Could you check a few things on this model? Use its own coordinates, in mm. A direction names the side the tool comes from. Round coordinates to 2 decimals unless told otherwise and drop trailing zeros. Order: outer loops, then holes, each group sorted by start corner. A loop starts at its lowest first (then second) coordinate and runs counter-clockwise, first axis right, second up. Notation, with made-up numbers: (74.5, 89) - (87.5, 89) arc R21 cw to (87.5, 124) - close; hole circle Ø4 at (25.25, 54.25). An arc over 180 degrees is marked (long way). Use one line per item in the form item = value.
from build123d import *

# Parameters (mm, degrees)
BOSS_EXTRUDE1_DEPTH = 26
FILLET1_R           = 2.5
CUT_EXTRUDE1_REACH  = 76.051
SKETCH2_R           = 3
CUT_EXTRUDE2_REACH  = 73.261
SKETCH3_R           = 3
CUT_EXTRUDE3_REACH  = 90.154
SKETCH4_R           = 3
SKETCH4_W           = 12
SKETCH4_H           = 20
BOSS_EXTRUDE2_DEPTH = 3
FILLET2_R           = 3.5


with BuildPart() as part:
    # Sketch1 → Boss-Extrude1 (new body)
    with BuildSketch(Plane(origin=(0, 0, 0), x_dir=(1, 0, 0), z_dir=(0, 1, 0))):
        Polygon((-55.080799194, 36.198206666), (23.167912006, 36.198206666), (-15.956443594, -31.567165046), align=None)
        Polygon((-51.616697579, 34.198206666), (19.703810391, 34.198206666), (-15.956443594, -27.567165046), align=None, mode=Mode.SUBTRACT)
    extrude(amount=BOSS_EXTRUDE1_DEPTH)

    # Fillet1
    fillet1_edges = [part.edges().sort_by_distance(p)[0] for p in [
        (-51.616697579, 13, -34.198206666),
        (-15.956443594, 13, 27.567165046),
        (19.703810391, 13, -34.198206666),
        (-55.080799194, 13, -36.198206666),
        (23.167912006, 13, -36.198206666),
        (-15.956443594, 13, 31.567165046),
    ]]
    fillet(fillet1_edges, radius=FILLET1_R)

    # Sketch2 → Cut-Extrude1 (cut, up to next)
    with BuildSketch(Plane(origin=(-25.636316123, 0, 14.801134015), x_dir=(0.49999999999999806, 0, 0.8660254037844397), z_dir=(-0.8660254037844397, 0, 0.49999999999999806)), mode=Mode.PRIVATE) as cut_extrude1_sk1:
        Polygon((3.632503749, 4.258248906), (-8.367496251, 8.741751094), (-8.367496251, 3), (3.632503749, 3), align=None)
    cut_extrude1_tool1 = extrude(cut_extrude1_sk1.sketch, amount=-CUT_EXTRUDE1_REACH, mode=Mode.PRIVATE) & part.part
    # Sketch2 → Cut-Extrude1 (cut, up to next)
    with BuildSketch(Plane(origin=(-25.636316123, 0, 14.801134015), x_dir=(0.49999999999999806, 0, 0.8660254037844397), z_dir=(-0.8660254037844397, 0, 0.49999999999999806)), mode=Mode.PRIVATE) as cut_extrude1_sk2:
        Polygon((-8.367496251, 13), (-8.367496251, 8.741751094), (3.632503749, 4.258248906), (3.632503749, 13), align=None)
    cut_extrude1_tool2 = extrude(cut_extrude1_sk2.sketch, amount=-CUT_EXTRUDE1_REACH, mode=Mode.PRIVATE) & part.part
    # Sketch2 → Cut-Extrude1 (cut, up to next)
    with BuildSketch(Plane(origin=(-25.636316123, 0, 14.801134015), x_dir=(0.49999999999999806, 0, 0.8660254037844397), z_dir=(-0.8660254037844397, 0, 0.49999999999999806)), mode=Mode.PRIVATE) as cut_extrude1_sk3:
        Polygon((3.632503749, 21.741751094), (-8.367496251, 17.258248906), (-8.367496251, 13), (3.632503749, 13), align=None)
    cut_extrude1_tool3 = extrude(cut_extrude1_sk3.sketch, amount=-CUT_EXTRUDE1_REACH, mode=Mode.PRIVATE) & part.part
    # Sketch2 → Cut-Extrude1 (cut, up to next)
    with BuildSketch(Plane(origin=(-25.636316123, 0, 14.801134015), x_dir=(0.49999999999999806, 0, 0.8660254037844397), z_dir=(-0.8660254037844397, 0, 0.49999999999999806)), mode=Mode.PRIVATE) as cut_extrude1_sk4:
        Polygon((-8.367496251, 23), (-8.367496251, 17.258248906), (3.632503749, 21.741751094), (3.632503749, 23), align=None)
    cut_extrude1_tool4 = extrude(cut_extrude1_sk4.sketch, amount=-CUT_EXTRUDE1_REACH, mode=Mode.PRIVATE) & part.part
    # Sketch2 → Cut-Extrude1 (cut, up to next)
    with BuildSketch(Plane(origin=(-25.636316123, 0, 14.801134015), x_dir=(0.49999999999999806, 0, 0.8660254037844397), z_dir=(-0.8660254037844397, 0, 0.49999999999999806)), mode=Mode.PRIVATE) as cut_extrude1_sk5:
        with Locations((-37.161724832, 13)):
            Circle(SKETCH2_R)
    cut_extrude1_tool5 = extrude(cut_extrude1_sk5.sketch, amount=-CUT_EXTRUDE1_REACH, mode=Mode.PRIVATE) & part.part
    add(cut_extrude1_tool1.solids().sort_by_distance((-27.460565, 4.989307, 11.641443))[0], mode=Mode.SUBTRACT)
    add(cut_extrude1_tool2.solids().sort_by_distance((-26.475179, 9.621142, 13.34818))[0], mode=Mode.SUBTRACT)
    add(cut_extrude1_tool3.solids().sort_by_distance((-26.475179, 16.378858, 13.34818))[0], mode=Mode.SUBTRACT)
    add(cut_extrude1_tool4.solids().sort_by_distance((-27.460565, 21.010693, 11.641443))[0], mode=Mode.SUBTRACT)
    add(cut_extrude1_tool5.solids().sort_by_distance((-44.217179, 13, -17.381864))[0], mode=Mode.SUBTRACT)

    # Sketch3 → Cut-Extrude2 (cut, up to next)
    with BuildSketch(Plane(origin=(1.701650732, 0, 0.982448508), x_dir=(0.5000000000000041, 0, -0.8660254037844364), z_dir=(0.8660254037844364, 0, 0.5000000000000041)), mode=Mode.PRIVATE) as cut_extrude2_sk1:
        Polygon((15.205281238, 13), (15.205281238, 8.741751094), (27.205281238, 4.258248906), (27.205281238, 13), align=None)
    cut_extrude2_tool1 = extrude(cut_extrude2_sk1.sketch, amount=-CUT_EXTRUDE2_REACH, mode=Mode.PRIVATE) & part.part
    # Sketch3 → Cut-Extrude2 (cut, up to next)
    with BuildSketch(Plane(origin=(1.701650732, 0, 0.982448508), x_dir=(0.5000000000000041, 0, -0.8660254037844364), z_dir=(0.8660254037844364, 0, 0.5000000000000041)), mode=Mode.PRIVATE) as cut_extrude2_sk2:
        Polygon((27.205281238, 4.258248906), (15.205281238, 8.741751094), (15.205281238, 3), (27.205281238, 3), align=None)
    cut_extrude2_tool2 = extrude(cut_extrude2_sk2.sketch, amount=-CUT_EXTRUDE2_REACH, mode=Mode.PRIVATE) & part.part
    # Sketch3 → Cut-Extrude2 (cut, up to next)
    with BuildSketch(Plane(origin=(1.701650732, 0, 0.982448508), x_dir=(0.5000000000000041, 0, -0.8660254037844364), z_dir=(0.8660254037844364, 0, 0.5000000000000041)), mode=Mode.PRIVATE) as cut_extrude2_sk3:
        Polygon((27.205281238, 21.741751094), (15.205281238, 17.258248906), (15.205281238, 13), (27.205281238, 13), align=None)
    cut_extrude2_tool3 = extrude(cut_extrude2_sk3.sketch, amount=-CUT_EXTRUDE2_REACH, mode=Mode.PRIVATE) & part.part
    # Sketch3 → Cut-Extrude2 (cut, up to next)
    with BuildSketch(Plane(origin=(1.701650732, 0, 0.982448508), x_dir=(0.5000000000000041, 0, -0.8660254037844364), z_dir=(0.8660254037844364, 0, 0.5000000000000041)), mode=Mode.PRIVATE) as cut_extrude2_sk4:
        Polygon((15.205281238, 23), (15.205281238, 17.258248906), (27.205281238, 21.741751094), (27.205281238, 23), align=None)
    cut_extrude2_tool4 = extrude(cut_extrude2_sk4.sketch, amount=-CUT_EXTRUDE2_REACH, mode=Mode.PRIVATE) & part.part
    # Sketch3 → Cut-Extrude2 (cut, up to next)
    with BuildSketch(Plane(origin=(1.701650732, 0, 0.982448508), x_dir=(0.5000000000000041, 0, -0.8660254037844364), z_dir=(0.8660254037844364, 0, 0.5000000000000041)), mode=Mode.PRIVATE) as cut_extrude2_sk5:
        with Locations((-13.588947343, 13)):
            Circle(SKETCH3_R)
    cut_extrude2_tool5 = extrude(cut_extrude2_sk5.sketch, amount=-CUT_EXTRUDE2_REACH, mode=Mode.PRIVATE) & part.part
    add(cut_extrude2_tool1.solids().sort_by_distance((12.649176, 9.621142, -17.979222))[0], mode=Mode.SUBTRACT)
    add(cut_extrude2_tool2.solids().sort_by_distance((11.663791, 4.989307, -16.272485))[0], mode=Mode.SUBTRACT)
    add(cut_extrude2_tool3.solids().sort_by_distance((12.649176, 16.378858, -17.979222))[0], mode=Mode.SUBTRACT)
    add(cut_extrude2_tool4.solids().sort_by_distance((11.663791, 21.010693, -16.272485))[0], mode=Mode.SUBTRACT)
    add(cut_extrude2_tool5.solids().sort_by_distance((-5.092823, 13, 12.750822))[0], mode=Mode.SUBTRACT)

    # Sketch4 → Cut-Extrude3 (cut, up to next)
    with BuildSketch(Plane(origin=(0, 0, -36.198206666), x_dir=(-1, 0, 0), z_dir=(0, 0, -1)), mode=Mode.PRIVATE) as cut_extrude3_sk1:
        with Locations((-1.440670696, 13)):
            Circle(SKETCH4_R)
    cut_extrude3_tool1 = extrude(cut_extrude3_sk1.sketch, amount=-CUT_EXTRUDE3_REACH, mode=Mode.PRIVATE) & part.part
    # Sketch4 → Cut-Extrude3 (cut, up to next)
    with BuildSketch(Plane(origin=(0, 0, -36.198206666), x_dir=(-1, 0, 0), z_dir=(0, 0, -1)), mode=Mode.PRIVATE) as cut_extrude3_sk2:
        with Locations((15.956443594, 13)):
            Rectangle(SKETCH4_W, SKETCH4_H)
    cut_extrude3_tool2 = extrude(cut_extrude3_sk2.sketch, amount=-CUT_EXTRUDE3_REACH, mode=Mode.PRIVATE) & part.part
    # Sketch4 → Cut-Extrude3 (cut, up to next)
    with BuildSketch(Plane(origin=(0, 0, -36.198206666), x_dir=(-1, 0, 0), z_dir=(0, 0, -1)), mode=Mode.PRIVATE) as cut_extrude3_sk3:
        with Locations((33.353557885, 13)):
            Rectangle(SKETCH4_W, SKETCH4_H)
    cut_extrude3_tool3 = extrude(cut_extrude3_sk3.sketch, amount=-CUT_EXTRUDE3_REACH, mode=Mode.PRIVATE) & part.part
    add(cut_extrude3_tool1.solids().sort_by_distance((1.440671, 13, -36.198207))[0], mode=Mode.SUBTRACT)
    add(cut_extrude3_tool2.solids().sort_by_distance((-15.956444, 13, -36.198207))[0], mode=Mode.SUBTRACT)
    add(cut_extrude3_tool3.solids().sort_by_distance((-33.353558, 13, -36.198207))[0], mode=Mode.SUBTRACT)

    # Sketch5 → Boss-Extrude2 (add)
    with BuildSketch(Plane.XZ):
        with BuildLine():
            Line((-17.038975349, -12.984749429), (-33.786570587, -3.31552081))
            Line((-33.786570587, -3.31552081), (-34.786570587, -5.047571617))
            Line((-34.786570587, -5.047571617), (-17.956443594, -14.764449967))
            Line((-17.956443594, -14.764449967), (-17.956443594, -34.198206666))
            Line((-17.956443594, -34.198206666), (-15.956443594, -34.198206666))
            Line((-15.956443594, -34.198206666), (-15.956443594, -14.859749429))
            ThreePointArc((-15.956443594, -14.859749429), (-17.038975349, -14.234749429), (-17.038975349, -12.984749429))
        make_face()
        with BuildLine():
            Line((-32.786570587, -1.583470002), (-33.786570587, -3.31552081))
            Line((-33.786570587, -3.31552081), (-17.038975349, -12.984749429))
            ThreePointArc((-17.038975349, -12.984749429), (-15.956443594, -12.359749429), (-14.873911839, -12.984749429))
            Line((-14.873911839, -12.984749429), (1.873683398, -3.31552081))
            Line((1.873683398, -3.31552081), (0.873683398, -1.583470002))
            Line((0.873683398, -1.583470002), (-15.956443594, -11.300348352))
            Line((-15.956443594, -11.300348352), (-32.786570587, -1.583470002))
        make_face()
        with BuildLine():
            Line((1.873683398, -3.31552081), (-14.873911839, -12.984749429))
            ThreePointArc((-14.873911839, -12.984749429), (-14.749036311, -13.286225622), (-14.706443594, -13.609749429))
            ThreePointArc((-14.706443594, -13.609749429), (-15.072560118, -14.493632905), (-15.956443594, -14.859749429))
            Line((-15.956443594, -14.859749429), (-15.956443594, -34.198206666))
            Line((-15.956443594, -34.198206666), (-13.956443594, -34.198206666))
            Line((-13.956443594, -34.198206666), (-13.956443594, -14.764449967))
            Line((-13.956443594, -14.764449967), (2.873683398, -5.047571617))
            Line((2.873683398, -5.047571617), (1.873683398, -3.31552081))
        make_face()
    extrude(amount=-BOSS_EXTRUDE2_DEPTH)

    # Fillet2
    fillet2_edges = [part.edges().sort_by_distance(p)[0] for p in [
        (0.873683398, 1.5, -1.583470002),
        (2.873683398, 1.5, -5.047571617),
        (-13.956443594, 1.5, -14.764449967),
        (-13.956443594, 1.5, -34.198206666),
        (-17.956443594, 1.5, -34.198206666),
        (-17.956443594, 1.5, -14.764449967),
        (-34.786570587, 1.5, -5.047571617),
        (-32.786570587, 1.5, -1.583470002),
        (-15.956443594, 1.5, -11.300348352),
    ]]
    fillet(fillet2_edges, radius=FILLET2_R)


solid = part.part
Item 1: If we mould it in two halves opening along X, with no side actions, what happens to faces 1 (the face through (-16, 0, -16)), 2 (the face through (-15.993, 13.182, 29.067)), 3 (the face through (17.52, 13.18, -32.98))? For each: released by +X, released by -X, zero draft, split by the parting line, or undercut.
Found:
face_1 = zero draft
face_2 = split by the parting line
face_3 = undercut
Item 2: For faces 4 (the face through (-22.966, 12.86, 17.454)), 5 (the face through (-21.956, 13, -35)), 6 (the face through (-34.45, 1.52, -6.46)), which set-ups out of +Z, -Z, +X, -X, +Y, -Y let a thin tool reach every point of the face, with its end or its side?
Found:
face_4 = -X
face_5 = -Z
face_6 = +Y, -Y
Item 3: Imagine slicing it at B-B on x = -37.5. Please give me the cut outline in (y, z).
Found:
outline = (0, -36.2) - (3, -36.2) - (3, -34.2) - (0, -34.2) - close; (0, -9.75) - (26, -9.75) - (26, -5.75) - (0, -5.75) - close; (23, -36.2) - (26, -36.2) - (26, -34.2) - (23, -34.2) - close
Item 4: Will these pins go through, and if not, where does the flat tip stop? P1, Ø3.5, axis at y = 1, z = -25.5, coming from the +X side; P2, Ø1, axis at y = 19, z = -21.5, coming from the -X side; P3, Ø0.9, axis at y = 2, z = -26.5, coming from the -X side; P4, Ø0.6, axis at x = -32.5, z = -35, coming from the -Y side.
Found:
P1 = 18
P2 = -46.88
P3 = -49.74
P4 = 0
Item 5: Imagine slicing it at A-A on y = 21.25. Please give me the cut outline in (x, z), plus the area to 3 significant figures.
Found:
outline = (-52.92, -32.45) arc R2.5 ccw to (-50.75, -36.2) - (-39.35, -36.2) - (-39.35, -34.2) - (-47.29, -34.2) arc R2.5 cw to (-49.45, -30.45) - (-28.09, 6.55) - (-29.82, 7.55) - close; (-27.35, -36.2) - (-21.96, -36.2) - (-21.96, -34.2) - (-27.35, -34.2) - close; (-23.82, 17.95) - (-22.09, 16.95) - (-18.12, 23.82) arc R2.5 cw to (-13.79, 23.82) - (7.57, -13.19) - (9.3, -12.19) - (-13.79, 27.82) arc R2.5 ccw to (-18.12, 27.82) - close; (-9.96, -36.2) - (18.84, -36.2) arc R2.5 ccw to (21, -32.45) - (15.3, -22.58) - (13.57, -23.58) - (17.54, -30.45) arc R2.5 cw to (15.37, -34.2) - (-9.96, -34.2) - close
area = 353 mm2
Item 6: I need wall thicknesses on L1, parallel to Z at x = -39, y = 8.5; L2, parallel to Z at x = 9, y = 11.25; L3, parallel to Z at x = -23.5, y = 4.75. Which ranges of each line are inside material? Lowest first, please.
Found:
L1 = -12.35 to -8.35
L2 = -36.2 to -34.2, -12.36 to -11.66
L3 = -36.2 to -34.2, 17.76 to 18.5
Item 7: Imagine slicing it at C-C on y = 13. State how many separate pieces and enclosed holes the cut face has, plus the area to 3 significant figures.
Found:
separate_pieces = 7
enclosed_holes = 0
area = 317 mm2
